```python
from build123d import *

# Parameters (mm, degrees)
F0_W     = 600
F0_H     = 500
F1_DEPTH = 31.473145
F3_DEPTH = 500


with BuildPart() as f1:
    # F0 (on Top) → F1 (new body)
    with BuildSketch(Plane.XY):
        with BuildLine():
            Line((-300, -250), (-300, 250))
            Line((-300, 250), (-400, 250))
            ThreePointArc((-400, 250), (-650, 0), (-400, -250))
            Line((-400, -250), (-300, -250))
        make_face()
        Rectangle(F0_W, F0_H)
        with BuildLine():
            Line((400, 250), (300, 250))
            Line((300, 250), (300, -250))
            Line((300, -250), (400, -250))
            ThreePointArc((400, -250), (650, 0), (400, 250))
        make_face()
    extrude(amount=F1_DEPTH)

    # F2 (on Top) → F3 (join)
    with BuildSketch(Plane.XY):
        with BuildLine():
            ThreePointArc((-280.5, 0), (-286.211418, 13.788582), (-300, 19.5))
            Line((-300, 19.5), (-300, -19.5))
            ThreePointArc((-300, -19.5), (-286.211418, -13.788582), (-280.5, 0))
        make_face()
        with BuildLine():
            Line((-300, -19.5), (-300, 19.5))
            ThreePointArc((-300, 19.5), (-319.5, 0), (-300, -19.5))
        make_face()
        with BuildLine():
            ThreePointArc((319.5, 0), (313.788582, 13.788582), (300, 19.5))
            Line((300, 19.5), (300, -19.5))
            ThreePointArc((300, -19.5), (313.788582, -13.788582), (319.5, 0))
        make_face()
        with BuildLine():
            Line((300, -19.5), (300, 19.5))
            ThreePointArc((300, 19.5), (280.5, 0), (300, -19.5))
        make_face()
    extrude(amount=-F3_DEPTH)


solid = f1.part
```
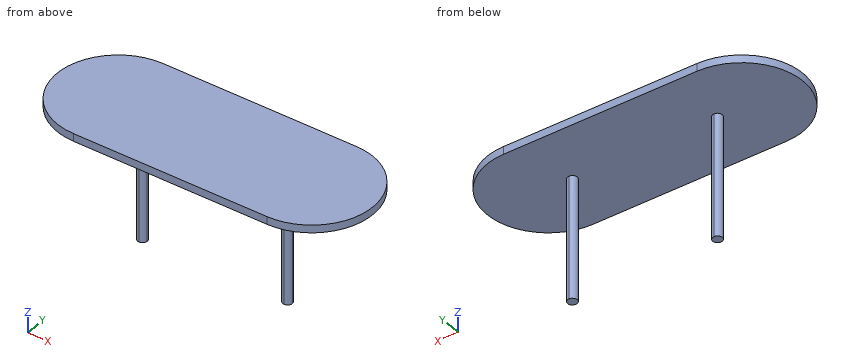
Here's how the part is built. I have some questions about the finished solid (model axes, mm). Round coordinates to 2 decimals unless told otherwise and drop trailing zeros. Order: outer loops, then holes, each group sorted by start corner. A loop starts at its lowest first (then second) coordinate and runs counter-clockwise, first axis right, second up. Notation, with made-up numbers: (76, 8) -> (119, 8) arc R20 cw to (119, 19) -> close; hole circle Ø10 at (22.25, -4). An arc over 180 degrees is marked (long way). Use a Markdown table: item, result. Add a question column.
(1) I need wall thicknesses on line 1 along Z through (x, y) = (381, -29). Which ranges of the line are inside material? Lowest first, please.
(2) For pin 1 Ø5 at (x, y) = (131, 98.5) entering from -Z, with a flat end and sliding along its axis, tell me the tip position at first contact or that it passes through.
(3) Suppose I cut it at B-B, the plane x = -166. Please give me the cut outline in (y, z).
(4) Suppose I cut it at A-A, the plane z = -375. Please give me the cut outline in (x, y).
(5) Suppose I cut it at C-C, the plane y = 113. Please give me the cut outline in (x, z), and give its area (3 significant figures).
Verdict:
| question | item | result |
|---|---|---|
| 1 | line 1 | 0 to 31.47 |
| 2 | pin 1 | z = 0 |
| 3 | outline | (-250, 0) -> (250, 0) -> (250, 31.47) -> (-250, 31.47) -> close |
| 4 | outline | circle Ø39 at (-300, 0); circle Ø39 at (300, 0) |
| 5 | outline | (-623, 0) -> (623, 0) -> (623, 31.47) -> (-623, 31.47) -> close |
| 5 | area | 39,200 mm2 |
